Read the model definition and answer for the solid it produces. Units are mm, in the model's axes. A direction names the side the tool comes from. Give positions to 0.01 mm unless a question says otherwise; leave off trailing zeros. Order: outer loops, then holes, each group sorted by start corner. A loop starts at its lowest first (then second) coordinate and runs counter-clockwise, first axis right, second up.
Item 1: Given pin 1 Ø1.5 at (x, y) = (132.5, -2) entering from -Z, flat-ended and moving along its own axis, determine where the tip first touches the part or whether it passes through.
Item 2: Which of the six approach directions +Z, -Z, +X, -X, +Y, -Y give full straight-line access (tool end or side, diameter ignored) to faces 3 (the face through (155.49, -1.48, 15.72)), 4 (the face through (261, 0, 228))?
Item 3: The mould has two halves that part along X. Classify faces 1 (the face through (114.28, -1.48, 15.49)), 2 (the face through (261, -3, 228)): +X half, -X half, draft (parallel to the pull), parting line (faces both ways), or undercut.
Item 4: Find the intervals of material crossed by line 1 along X through (y, z) = (-0.7, 215); line 2 along Z through (x, y) = (18, -1.8); line 3 along X through (y, z) = (-1.95, 435), in increasing order.
Item 5: A cutting plane is placed at A-A (x = 152). Write down the section's boundary in (y, z), plus the area to 3 significant figures.
from build123d import *

# Parameters (mm, degrees)
F0_R     = 3
F1_DEPTH = 3


with BuildPart() as f1:
    # F0 (on Front) → F1 (new body)
    with BuildSketch(Plane.XZ):
        with BuildLine():
            Line((0, 450), (0, 0))
            Line((0, 0), (110, 0))
            Line((110, 0), (110, 5))
            ThreePointArc((110, 5), (114.393398, 15.606602), (125, 20))
            Line((125, 20), (145, 20))
            ThreePointArc((145, 20), (155.606602, 15.606602), (160, 5))
            Line((160, 5), (160, 0))
            Line((160, 0), (530, 0))
            Line((530, 0), (530, 450))
            Line((530, 450), (0, 450))
        make_face()
        with Locations((18, 15)):
            Circle(F0_R, mode=Mode.SUBTRACT)
        with Locations((18, 215)):
            Circle(F0_R, mode=Mode.SUBTRACT)
        with Locations((512, 15)):
            Circle(F0_R, mode=Mode.SUBTRACT)
        with Locations((512, 215)):
            Circle(F0_R, mode=Mode.SUBTRACT)
        with Locations((18, 235)):
            Circle(F0_R, mode=Mode.SUBTRACT)
        with Locations((18, 435)):
            Circle(F0_R, mode=Mode.SUBTRACT)
        with Locations((255, 435)):
            Circle(F0_R, mode=Mode.SUBTRACT)
        with Locations((512, 235)):
            Circle(F0_R, mode=Mode.SUBTRACT)
        with Locations((275, 435)):
            Circle(F0_R, mode=Mode.SUBTRACT)
        with Locations((512, 435)):
            Circle(F0_R, mode=Mode.SUBTRACT)
    extrude(amount=F1_DEPTH)


solid = f1.part
Response values:
1. pin 1: stops at z = 20
2. face 3: -Z, +Y, -Y
2. face 4: +Z, -Z, +X, -X, +Y
3. face 1: undercut
3. face 2: draft
4. line 1: x = 0 to 15, 21 to 509, 515 to 530
4. line 2: z = 0 to 12, 18 to 212, 218 to 232, 238 to 432, 438 to 450
4. line 3: x = 0 to 15, 21 to 252, 258 to 272, 278 to 509, 515 to 530
5. outline: (-3, 18.27) - (0, 18.27) - (0, 450) - (-3, 450) - close
5. area: 1,300 mm2
